Input: part model. Units: mm. Frame: model coordinates. Give positions to 0.01 mm unless a question says otherwise; leave off trailing zeros. Write each loop counter-clockwise with the first axis right and the second up, starting at its lowest first coordinate (ties: lowest second). Pieces come first, ordered by that corner, then holes.
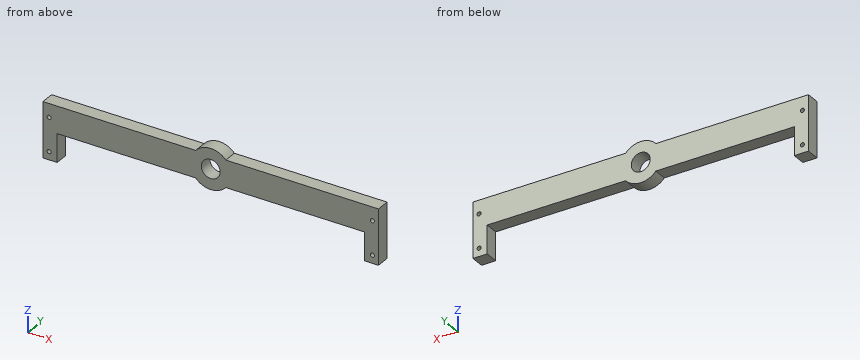
```python
from build123d import *

# Parameters (mm, degrees)
SKETCH1_R           = 1.5
SKETCH1_R_2         = 6.975
BOSS_EXTRUDE1_DEPTH = 10


with BuildPart() as part:
    # Sketch1 → Boss-Extrude1 (new body)
    with BuildSketch(Plane(origin=(0, 0, 0), x_dir=(1, 0, 0), z_dir=(0, 1, 0))):
        with BuildLine():
            Line((-124, -10), (-11.180339887, -10))
            ThreePointArc((-11.180339887, -10), (0, -15), (11.180339887, -10))
            Line((11.180339887, -10), (124, -10))
            Line((124, -10), (124, 10))
            Line((124, 10), (124, 31))
            Line((124, 31), (113.5, 31))
            Line((113.5, 31), (113.5, 10))
            Line((113.5, 10), (11.180339887, 10))
            ThreePointArc((11.180339887, 10), (0, 15), (-11.180339887, 10))
            Line((-11.180339887, 10), (-113.5, 10))
            Line((-113.5, 10), (-113.5, 31))
            Line((-113.5, 31), (-124, 31))
            Line((-124, 31), (-124, 10))
            Line((-124, 10), (-124, -10))
        make_face()
        with Locations(Location((-119.5, 0, 0), (0, 0, 270))):
            Circle(SKETCH1_R, mode=Mode.SUBTRACT)
        with Locations(Location((119.5, 0, 0), (0, 0, 90))):
            Circle(SKETCH1_R, mode=Mode.SUBTRACT)
        with Locations(Location((0, 0, 0), (0, 0, 270))):
            Circle(SKETCH1_R_2, mode=Mode.SUBTRACT)
        with Locations(Location((-119.5, 25, 0), (0, 0, 270))):
            Circle(SKETCH1_R, mode=Mode.SUBTRACT)
        with Locations(Location((119.5, 25, 0), (0, 0, 90))):
            Circle(SKETCH1_R, mode=Mode.SUBTRACT)
    extrude(amount=BOSS_EXTRUDE1_DEPTH)


solid = part.part
```
Q1. Pin query (flat end, axial travel): pin 1 (5 mm diameter, centred on x = 91, y = 3.5, fed in from +Z); pin 2 (3 mm diameter, centred on x = 68.5, y = 6, fed in from -Z). Return the tip coordinate at first contact, or that it passes through.
Q2. Section D-D, the plane x = -33.5. Return the cut outline in (y, z), then the cut area to 3 significant figures.
Q3. Section A-A, the plane x = 0. Return the cut outline in (y, z) (3 decimals), then the cut area to 4 significant figures.
Q4. Section B-B, the plane z = -18.5. Return the cut outline in (x, y), then the cut area to 3 significant figures.
Q5. Material intervals for line 1 along X through (y, z) = (7.5, 0) (3 decimals); line 2 along X through (y, z) = (2.25, -25); line 3 along Z through (x, y) = (119.5, 5.25), sorted ascending.
Q6. Section C-C, the plane y = 3.25. Return the cut outline in (x, z) (3 decimals).
Solutions:
1. pin 1: stops at z = 10
1. pin 2: stops at z = -10
2. outline: (0, -10) - (10, -10) - (10, 10) - (0, 10) - close
2. area: 200 mm2
3. outline: (0, -15) - (10, -15) - (10, -6.975) - (0, -6.975) - close; (0, 6.975) - (10, 6.975) - (10, 15) - (0, 15) - close
3. area: 160.5 mm2
4. outline: (-124, 0) - (-113.5, 0) - (-113.5, 10) - (-124, 10) - close; (113.5, 0) - (124, 0) - (124, 10) - (113.5, 10) - close
4. area: 210 mm2
5. line 1: x = -124 to -121, -118 to -6.975, 6.975 to 118, 121 to 124
5. line 2: x = -124 to -121, -118 to -113.5, 113.5 to 118, 121 to 124
5. line 3: z = -31 to -26.5, -23.5 to -1.5, 1.5 to 10
6. outline: (-124, -31) - (-113.5, -31) - (-113.5, -10) - (-11.18, -10) arc R15 ccw to (11.18, -10) - (113.5, -10) - (113.5, -31) - (124, -31) - (124, 10) - (11.18, 10) arc R15 ccw to (-11.18, 10) - (-124, 10) - close; hole circle Ø3 at (-119.5, -25); hole circle Ø3 at (-119.5, 0); hole circle Ø13.95 at (0, 0); hole circle Ø3 at (119.5, -25); hole circle Ø3 at (119.5, 0)
